The listing builds one solid part. Answer for the finished solid, in the listing's coordinates (mm). Face numbers are marked on the shaded views. A direction names the side the tool comes from. Coordinates: 2 decimals unless noted, no trailing zeros. Write each loop counter-clockwise with the first axis right and the second up, starting at its lowest first coordinate (ties: lowest second). Pieces come first, ordered by that corner, then holes. Notation, with made-up numbers: M 22,-15.5 L 65,-15.5 A23 ccw 65,18.5 Z; hole C -2,46 d11. An arc over 180 degrees is marked long. Put each result on its own line as item: value. Start each with the question number.
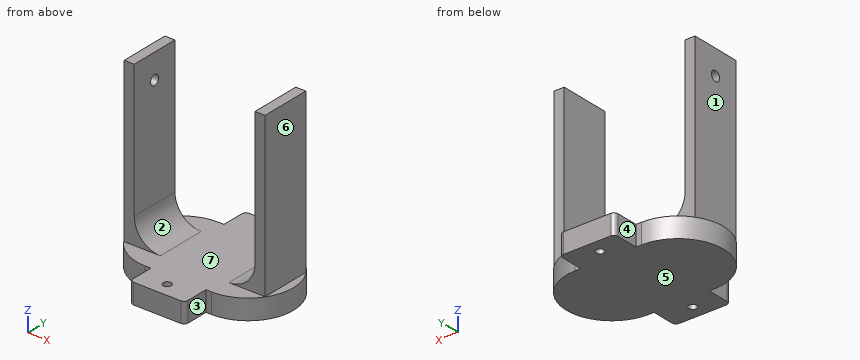
```python
from build123d import *

# Parameters (mm, degrees)
SKETCH_1_R          = 2
EXTRUDE_1_DEPTH     = 10
SKETCH_2_W          = 5
SKETCH_2_H          = 25
EXTRUDE_2_DEPTH     = 80
EXTRUDE_3_DEPTH     = 25
EXTRUDE_4_DEPTH     = 25
CUT_EXTRUDE_1_REACH = 124.376
SKETCH_8_R          = 2.5


with BuildPart() as part:
    # 草圖1 → 填料-伸長1 (new body)
    # profile 1 of 3: a face of its own
    with BuildSketch(Plane.XY):
        with BuildLine():
            Line((-12.867229619, 32.988964319), (20.132770381, 32.988964319))
            ThreePointArc((20.132770381, 32.988964319), (42.632770381, 10.488964319), (20.132770381, -12.011035681))
            Line((20.132770381, -12.011035681), (-12.867229619, -12.011035681))
            ThreePointArc((-12.867229619, -12.011035681), (-35.367229619, 10.488964319), (-12.867229619, 32.988964319))
        make_face()
    # profile 2 of 3: a face of its own
    with BuildSketch(Plane.XY):
        with BuildLine():
            Line((-10.067229619, 32.988964319), (17.332770381, 32.988964319))
            Line((17.332770381, 32.988964319), (17.332770381, 43.988964319))
            ThreePointArc((17.332770381, 43.988964319), (16.746983944, 45.403177881), (15.332770381, 45.988964319))
            Line((15.332770381, 45.988964319), (-8.067229619, 45.988964319))
            ThreePointArc((-8.067229619, 45.988964319), (-9.481443181, 45.403177881), (-10.067229619, 43.988964319))
            Line((-10.067229619, 43.988964319), (-10.067229619, 32.988964319))
        make_face()
        with Locations((2.921464597, 38.988964319)):
            Circle(SKETCH_1_R, mode=Mode.SUBTRACT)
    # profile 3 of 3: a face of its own
    with BuildSketch(Plane.XY):
        with BuildLine():
            Line((-10.067229619, -12.011035681), (17.332770381, -12.011035681))
            Line((17.332770381, -12.011035681), (17.332770381, -23.011035681))
            ThreePointArc((17.332770381, -23.011035681), (16.746983944, -24.425249243), (15.332770381, -25.011035681))
            Line((15.332770381, -25.011035681), (-8.067229619, -25.011035681))
            ThreePointArc((-8.067229619, -25.011035681), (-9.481443181, -24.425249243), (-10.067229619, -23.011035681))
            Line((-10.067229619, -23.011035681), (-10.067229619, -12.011035681))
        make_face()
        with Locations((2.921464597, -18.011035681)):
            Circle(SKETCH_1_R, mode=Mode.SUBTRACT)
    extrude(amount=EXTRUDE_1_DEPTH)

    # 草圖2 → 填料-伸長2 (add)
    with BuildSketch(Plane.XY.offset(10)):
        with Locations((-28.867229619, 10.488964319)):
            Rectangle(SKETCH_2_W, SKETCH_2_H)
        with Locations((36.132770381, 10.488964319)):
            Rectangle(SKETCH_2_W, SKETCH_2_H)
    extrude(amount=EXTRUDE_2_DEPTH)

    # 草圖6 → 填料-伸長3 (add)
    with BuildSketch(Plane.XZ.offset(2.011035681)):
        with BuildLine():
            ThreePointArc((-13.367229619, 10), (-22.559617774, 13.807611845), (-26.367229619, 23))
            Line((-26.367229619, 23), (-26.367229619, 10))
            Line((-26.367229619, 10), (-13.367229619, 10))
        make_face()
    extrude(amount=-EXTRUDE_3_DEPTH)

    # 草圖7 → 填料-伸長4 (add)
    with BuildSketch(Plane.XZ.offset(2.011035681)):
        with BuildLine():
            ThreePointArc((33.632770381, 23), (29.825158537, 13.807611845), (20.632770381, 10))
            Line((20.632770381, 10), (33.632770381, 10))
            Line((33.632770381, 10), (33.632770381, 23))
        make_face()
    extrude(amount=-EXTRUDE_4_DEPTH)

    # 草圖8 → 除料-伸長1 (cut, up to next)
    with BuildSketch(Plane(origin=(-26.367229619, 0, 0), x_dir=(0, 0, -1), z_dir=(1, 0, 0)), mode=Mode.PRIVATE) as cut_extrude_1_sk1:
        with Locations(Location((-77.7, 10.488964319, 0), (0, 0, 90))):
            Circle(SKETCH_8_R)
    cut_extrude_1_tool1 = extrude(cut_extrude_1_sk1.sketch, amount=-CUT_EXTRUDE_1_REACH, mode=Mode.PRIVATE) & part.part
    add(cut_extrude_1_tool1.solids().sort_by_distance((-26.36723, 10.488964, 77.7))[0], mode=Mode.SUBTRACT)


solid = part.part
```
1) For the marked faces 1, 2, 3 and 4, determine the directions among +Z, -Z, +X, -X, +Y, -Y from which every point of the face is accessible in a straight line to the end or side of a thin tool.
2) A cutting plane is placed at A-A on z = 35. Write down the section's boundary in (x, y), then the cut area to 3 significant figures.
3) A cutting plane is placed at D-D on y = 18. Write down the section's boundary in (x, z), then the cut area to 3 significant figures.
4) A cutting plane is placed at B-B on z = 77.7. Write down the section's boundary in (x, y).
5) Straight lines are drawn through the part: probe 1 along X at (y, z) = (4.5, 60); probe 2 along Z at (x, y) = (29, 29); probe 3 along X at (y, z) = (16, 14). For each, find the intervals that lie inside material, in ascending order.
6) A cutting plane is placed at C-C on x = 24. Write down the section's boundary in (y, z).
7) Given pin 1 Ø1.4 at (x, z) = (-11.5, 4.5) entering from +Y; pin 2 Ø1.4 at (x, z) = (-11, 4) entering from -Y; pin 3 Ø5 at (y, z) = (37, 4.5) entering from +X; pin 4 Ø10 at (y, z) = (-7.5, 74.5) entering from +X, each flat-ended and moving along its own axis, determine where each tip first touches the part or whether it passes through.
8) Determine the mould class of the marked faces 5, 6 and 7 for opening direction X: +X half, -X half, draft (parallel to the pull), parting line (faces both ways), or undercut.
Answers follow:
1. face 1: +Z, -X, +Y, -Y
1. face 2: +Z, +Y, -Y
1. face 3: +Z, -Z, +X, -Y
1. face 4: +Z, -Z, -X, +Y
2. outline: M -31.37,-2.01 L -26.37,-2.01 L -26.37,22.99 L -31.37,22.99 Z; M 33.63,-2.01 L 38.63,-2.01 L 38.63,22.99 L 33.63,22.99 Z
2. area: 250 mm²
3. outline: M -34.08,0 L 41.34,0 L 41.34,10 L 38.63,10 L 38.63,90 L 33.63,90 L 33.63,23 A13 cw 20.63,10 L -13.37,10 A13 cw -26.37,23 L -26.37,90 L -31.37,90 L -31.37,10 L -34.08,10 Z
3. area: 1,630 mm²
4. outline: M -31.37,-2.01 L -26.37,-2.01 L -26.37,7.99 L -31.37,7.99 Z; M -31.37,12.99 L -26.37,12.99 L -26.37,22.99 L -31.37,22.99 Z; M 33.63,-2.01 L 38.63,-2.01 L 38.63,22.99 L 33.63,22.99 Z
5. probe 1: x = -31.37 to -26.37, 33.63 to 38.63
5. probe 2: z = 0 to 10
5. probe 3: x = -31.37 to -22.75, 30.01 to 38.63
6. outline: M -11.68,0 L 32.65,0 L 32.65,10 L 22.99,10 L 22.99,10.44 L -2.01,10.44 L -2.01,10 L -11.68,10 Z
7. pin 1: stops at y = 32.99
7. pin 2: stops at y = -12.01
7. pin 3: stops at x = 17.33
7. pin 4: passes through
8. face 5: draft
8. face 6: +X half
8. face 7: undercut
